Work out the finished part from the listing and answer in its coordinate system (mm). A direction names the side the tool comes from. Round coordinates to 2 decimals unless told otherwise and drop trailing zeros. Order: outer loops, then holes, each group sorted by start corner. A loop starts at its lowest first (then second) coordinate and runs counter-clockwise, first axis right, second up. Notation, with made-up numbers: (15.5, -7.75) - (19.5, -7.75) arc R22 ccw to (19.5, 19.25) - close; hole circle Ø2 at (-6, 38.25). An arc over 180 degrees is marked (long way). Use one line per item in the form item = value. Start each with the question number.
Q1. For a pull along Z with two mould halves and no side action, classify faces 1 (the cylindrical face through (8.986, -3.513, -0.195)), 2 (the cylindrical face through (-9.014, -3.513, -0.195)), 3 (the cylindrical face through (-8.838, -3.407, 6.697)), 4 (the flat face through (2, 3, 0)) as +Z half, -Z half, draft (parallel to the pull), parting line (faces both ways), or undercut.
Q2. Given P1, Ø12, axis at x = 0, z = -7.5, coming from the -Y side; P2, Ø1, axis at x = -6.5, y = -5, coming from the -Z side, each flat-ended and moving along its own axis, determine where each tip first touches the part or whether it passes through.
Q3. Find the intervals of material crossed by line 1 (X direction, y = 3.8, z = 0); line 2 (X direction, y = -0.5, z = 3); line 3 (Y direction, x = 8.6, z = 0), in increasing order. Write a range as [from, to].
Q4. The part is cut by section C-C on x = 0. Determine the outline of the cut face in (y, z), plus the area to 3 significant figures.
Q5. Which of the six approach directions +Z, -Z, +X, -X, +Y, -Y give full straight-line access (tool end or side, diameter ignored) to faces 5 (the flat face through (8, -2, 0)), 6 (the flat face through (0, 4, 10))?
Q6. The part is cut by section A-A on y = -0.25. Determine the outline of the cut face in (x, z).
Q7. The part is cut by section B-B on z = 0. Determine the outline of the cut face in (x, y), plus the area to 3 significant figures.
Q8. The part is cut by section D-D on y = 4. Determine the outline of the cut face in (x, z), plus the area to 3 significant figures.
Autodesk Inventor part; units mm, degrees
ref_plane "YZ Plane" through (0, 0, 0) normal (1, 0, 0) x (0, 1, 0)
ref_plane "XZ Plane" through (0, 0, 0) normal (0, 1, 0) x (-1, 0, 0)
ref_plane "XY Plane" through (0, 0, 0) normal (0, 0, 1) x (1, 0, 0)
sketch "Sketch1" plane through (0, 0, 0) normal (0, 0, 1) x (1, 0, 0)
  line L0 (-10, 5) -> (10, 5)
  line L1 (10, 5) -> (10, -5)
  line L2 (10, -5) -> (-10, -5)
  line L3 (-10, -5) -> (-10, 5)
  line L4 (-10, 5) -> (10, -5) construction
  line L5 (10, 5) -> (-10, -5) construction
  point P0 (0, 0)
extrude "Extrusion1" add sketch "Sketch1" along normal mid plane 20
sketch "Sketch3" plane through (10, -5, 10) normal (1, 0, 0) x (0, 0, -1)
  point P0 (10, 5)
sketch "Sketch4" plane through (10, -5, 10) normal (1, 0, 0) x (0, 0, -1)
  line L0 (0, 0) -> (20, 0)
  arc A0 (5, 0) -> (15, 0) centre (10, 0) ccw
  point P0 (10, 5)
  dimension "d9" = 10
extrude "Extrusion3" add sketch "Sketch4" against normal up to surface (20 mm away)
sketch "Sketch2" plane through (0, 0, 10) normal (0, 0, 1) x (1, 0, 0)
  line L0 (-8, -16.4616) -> (8, -16.4616)
  line L1 (8, -16.4616) -> (8, 3)
  line L2 (8, 3) -> (-8, 3)
  line L3 (-8, 3) -> (-8, -16.4616)
  line L4 (-10, 5) -> (-10, -5)
  line L5 (10, -5) -> (10, 5)
  line L6 (10, 5) -> (-10, 5)
  point P0 (0, 0)
  dimension "d4" = 2
  dimension "d5" = 2
  dimension "d6" = 2
extrude "Extrusion2" cut sketch "Sketch2" against normal blind 30
sketch "Sketch5" plane through (10, -5, 10) normal (1, 0, 0) x (0, 0, -1)
  line L0 (0, 8) -> (0, 0)
  line L1 (5, 0) -> (0, 0)
  line L2 (0, 3) -> (5, 3)
  line L3 (5, 3) -> (5, 0)
  line L4 (5, 0) -> (0, 0)
  line L5 (0, 0) -> (0, 3)
  arc A0 (5, 0) -> (15, 0) centre (10, 0) ccw
  line L6 (20, 10) -> (20, 0)
  line L7 (15, 0) -> (20, 0)
  line L8 (20, 0) -> (20, 3)
  line L9 (20, 3) -> (15, 3)
  line L10 (15, 3) -> (15, 0)
  point P0 (10, 5)
  dimension "d12" = 3
extrude "Extrusion4" cut sketch "Sketch5" against normal blind 30
fillet "Fillet1" radius 6 4 edges at (9, -2, 5) (9, -2, -5) (-9, -2, 5) (-9, -2, -5)
chamfer "Chamfer1" distance 0.3 angle 45 12 edges at (0, 5, 10) (10, 5, 0) (0, 5, -10) (-10, 5, 0) (-10, 1.5, 10) (10, 1.5, 10) (10, 1.5, -10) (-10, 1.5, -10) (-10, -3.3741, 6.7351) (10, -3.3741, -6.7351) (10, -10, 0) (10, -3.3741, 6.7351)
sketch "Sketch6" plane through (-10, -4.2, -14.7) normal (-1, 0, 0) x (0, 0, 1)
  arc A0 (9.8858, -2.1504) -> (19.5142, -2.1504) centre (14.7, -0.8) ccw
  circle A1 centre (14.7, -0.8) radius 1.5
  point P0 (14.7, 4.2)
  dimension "d20" = 3
extrude "Extrusion5" cut sketch "Sketch6" against normal blind 30
sketch "Sketch7" plane through (-8, 3, 10) normal (0, -1, 0) x (1, 0, 0)
  point P0 (8, -10)
  point P1 (8, -10)
hole "Hole1" at (0, 3, 0) direction (0, 1, 0) diameter 3.5 depth 11.8 tip angle 118
properties part number "Ball Track Mounting Plate" material "Brass, Soft Yellow"
Found:
q1.face_1 = undercut
q1.face_2 = undercut
q1.face_3 = +Z half
q1.face_4 = draft
q2.P1 = 3
q2.P2 = through
q3.line_1 = [-10, -1.75], [1.75, 10]
q3.line_2 = [-10, -8], [8, 10]
q3.line_3 = [-10, -6.5], [-3.5, 5]
q4.outline = (3, -10) - (4.7, -10) - (5, -9.7) - (5, -1.75) - (3, -1.75) - close; (3, 1.75) - (5, 1.75) - (5, 9.7) - (4.7, 10) - (3, 10) - close
q4.area = 32.9 mm²
q5.face_5 = +Z, -Z, -Y
q5.face_6 = +Z, +X, -X, +Y, -Y
q6.outline = (-10, -9.7) - (-9.7, -10) - (-8, -10) - (-8, 10) - (-9.7, 10) - (-10, 9.7) - close; (8, -10) - (9.7, -10) - (10, -9.7) - (10, 9.7) - (9.7, 10) - (8, 10) - close
q7.outline = (-10, -9.7) - (-9.7, -10) - (-8, -10) - (-8, -6.5) - (-10, -6.5) - close; (-10, -3.5) - (-8, -3.5) - (-8, 3) - (-1.75, 3) - (-1.75, 5) - (-9.7, 5) - (-10, 4.7) - close; (1.75, 3) - (8, 3) - (8, -3.5) - (10, -3.5) - (10, 4.7) - (9.7, 5) - (1.75, 5) - close; (8, -10) - (9.7, -10) - (10, -9.7) - (10, -6.5) - (8, -6.5) - close
q7.area = 72.8 mm²
q8.outline = (-10, -9.7) - (-9.7, -10) - (9.7, -10) - (10, -9.7) - (10, 9.7) - (9.7, 10) - (-9.7, 10) - (-10, 9.7) - close; hole circle Ø3.5 at (0, 0)
q8.area = 390 mm²
